The model under review builds one solid part; all positions refer to its coordinate system, in mm. Round coordinates to 2 decimals unless told otherwise and drop trailing zeros. Loops run counter-clockwise (first coordinate to the right, second up) from the corner with the lowest first, then second, coordinate; pieces in that order, holes last. Notation, with made-up numbers: M 48,86 L 64,86 A32 cw 64,122 Z; hole C 12.5,48.25 d2. An arc over 180 degrees is marked long. One line per question, with ' | ' between items.
from build123d import *

# Parameters (mm, degrees)
SKETCH1_W           = 76.2
SKETCH1_H           = 266.7
SKETCH1_R           = 2.4892
BOSS_EXTRUDE1_DEPTH = 3.175
SKETCH2_R           = 11.1125
SKETCH2_R_2         = 3.2512
SKETCH2_R_3         = 3.175
SKETCH2_R_4         = 6.35
CUT_EXTRUDE1_DEPTH  = 3.175


with BuildPart() as part:
    # Sketch1 → Boss-Extrude1 (new body)
    with BuildSketch(Plane.XY):
        with Locations((38.1, -133.35)):
            Rectangle(SKETCH1_W, SKETCH1_H)
        with Locations((19.05, -6.35)):
            Circle(SKETCH1_R, mode=Mode.SUBTRACT)
        with Locations((57.15, -6.35)):
            Circle(SKETCH1_R, mode=Mode.SUBTRACT)
        with Locations((71.4375, -17.4625)):
            Circle(SKETCH1_R, mode=Mode.SUBTRACT)
        with Locations((4.7625, -17.4625)):
            Circle(SKETCH1_R, mode=Mode.SUBTRACT)
        with Locations((71.4375, -139.7)):
            Circle(SKETCH1_R, mode=Mode.SUBTRACT)
        with Locations((4.7625, -139.7)):
            Circle(SKETCH1_R, mode=Mode.SUBTRACT)
        with Locations((71.4375, -249.2375)):
            Circle(SKETCH1_R, mode=Mode.SUBTRACT)
        with Locations((4.7625, -249.2375)):
            Circle(SKETCH1_R, mode=Mode.SUBTRACT)
        with Locations((19.05, -260.35)):
            Circle(SKETCH1_R, mode=Mode.SUBTRACT)
        with Locations((57.15, -260.35)):
            Circle(SKETCH1_R, mode=Mode.SUBTRACT)
    extrude(amount=BOSS_EXTRUDE1_DEPTH)

    # Sketch2 → Cut-Extrude1 (cut)
    with BuildSketch(Plane.XY.offset(3.175)):
        with Locations((38.1, -104.775)):
            Circle(SKETCH2_R)
        with Locations((38.1, -174.625)):
            Circle(SKETCH2_R)
        with Locations((20.599908, -174.625)):
            Circle(SKETCH2_R_2)
        with Locations((20.599908, -104.775)):
            Circle(SKETCH2_R_2)
        with Locations((25.4, -234.95)):
            Circle(SKETCH2_R_3)
        with Locations((50.8, -234.95)):
            Circle(SKETCH2_R_3)
        with Locations((38.1, -44.45)):
            Circle(SKETCH2_R_4)
    extrude(amount=-CUT_EXTRUDE1_DEPTH, mode=Mode.SUBTRACT)


solid = part.part
1) Add section B-B on x = 57.15. State the section outline as (y, z) points (3 decimals), then the cut area to 3 significant figures.
Output values:
outline: M -266.7,0 L -262.839,0 L -262.839,3.175 L -266.7,3.175 Z; M -257.861,0 L -8.839,0 L -8.839,3.175 L -257.861,3.175 Z; M -3.861,0 L 0,0 L 0,3.175 L -3.861,3.175 Z | area: 815 mm²
2) Mouldability with a two-part tool opening along X and no side actions: class faces 1 (the flat face through (38, -131, 0)), 2 (the cylindrical face through (16.563, -6.241, 1.565)), 3 (the cylindrical face through (20.39, -258.25, 1.57)) as +X half, -X half, draft (parallel to the pull), parting line (faces both ways), or undercut.
Output values:
face 1: draft | face 2: undercut | face 3: undercut
3) For line 1 (X direction, y = -234.95, z = 1.1) (3 decimals); line 2 (Y direction, x = 38.1, z = 0.95); line 3 (X direction, y = -139.7, z = 0.65), list the stretches that pass through material, from the lowest coordinate up.
Output values:
line 1: x = 0 to 22.225, 28.575 to 47.625, 53.975 to 76.2 | line 2: y = -266.7 to -185.74, -163.51 to -115.89, -93.66 to -50.8, -38.1 to 0 | line 3: x = 0 to 2.27, 7.25 to 68.95, 73.93 to 76.2
4) Insertion check: P1, Ø3, axis at x = 4.76, y = -17.46, coming from the +Z side. The pin has a flat end and moves straight along its axis. Give the tip position at first contact, or say it passes through.
Output values:
P1: passes through
5) Add section D-D on y = -44.45. State the section outline as (x, z) points (3 decimals), then the cut area to 3 significant figures.
Output values:
outline: M 0,0 L 31.75,0 L 31.75,3.175 L 0,3.175 Z; M 44.45,0 L 76.2,0 L 76.2,3.175 L 44.45,3.175 Z | area: 202 mm²
6) Add section A-A on y = -260.35. State the section outline as (x, z) points (3 decimals).
Output values:
outline: M 0,0 L 16.561,0 L 16.561,3.175 L 0,3.175 Z; M 21.539,0 L 54.661,0 L 54.661,3.175 L 21.539,3.175 Z; M 59.639,0 L 76.2,0 L 76.2,3.175 L 59.639,3.175 Z
7) Add section C-C on x = 38.1. State the section outline as (y, z) points (1 decimal), then the cut area to 3 significant figures.
Output values:
outline: M -266.7,0 L -185.7,0 L -185.7,3.2 L -266.7,3.2 Z; M -163.5,0 L -115.9,0 L -115.9,3.2 L -163.5,3.2 Z; M -93.7,0 L -50.8,0 L -50.8,3.2 L -93.7,3.2 Z; M -38.1,0 L 0,0 L 0,3.2 L -38.1,3.2 Z | area: 665 mm²
